Work out the finished part from the listing and answer in its coordinate system (mm). A direction names the side the tool comes from. Round coordinates to 2 decimals unless told otherwise and drop trailing zeros. Write each loop counter-clockwise with the first axis right and the second up, starting at its lowest first coordinate (ties: lowest second). Pieces come first, ordered by that corner, then holes. Notation, with made-up numbers: (9, -21) - (48, -21) arc R20 cw to (48, 17) - close; hole circle Ø4 at (-5, -15). An arc over 180 degrees is marked (long way). Write item = value, one per line. Start each with the question number.
Autodesk Inventor part; units mm, degrees
ref_plane "YZ Plane" through (0, 0, 0) normal (1, 0, 0) x (0, 1, 0)
ref_plane "XZ Plane" through (0, 0, 0) normal (0, 1, 0) x (-1, 0, 0)
ref_plane "XY Plane" through (0, 0, 0) normal (0, 0, 1) x (1, 0, 0)
sketch "Sketch1" plane through (0, 0, 0) normal (1, 0, 0) x (0, 1, 0)
  line L0 (0, 0) -> (44.45, 0)
  line L1 (44.45, 0) -> (44.45, 92.075)
  line L2 (44.45, 92.075) -> (0, 92.075)
  line L3 (0, 92.075) -> (0, 0)
  line L4 (14.2875, 92.075) -> (14.2875, 0) construction
  line L5 (30.1625, 92.075) -> (30.1625, 0) construction
  line L6 (22.225, 92.075) -> (22.225, 0) construction
  circle A0 centre (34.925, 79.375) radius 4.7625 construction
  circle A1 centre (9.525, 12.7) radius 4.7625 construction
  circle A2 centre (34.925, 79.375) radius 7.1437
  circle A3 centre (9.525, 12.7) radius 7.1437
  line L7 (7.9375, 68.2625) -> (36.5125, 68.2625)
  line L8 (36.5125, 68.2625) -> (36.5125, 23.8125)
  line L9 (36.5125, 23.8125) -> (7.9375, 23.8125)
  line L10 (7.9375, 23.8125) -> (7.9375, 68.2625)
  line L11 (7.9375, 46.0375) -> (36.5125, 46.0375) construction
  circle A4 centre (6.0325, 79.375) radius 3.3782
  circle A5 centre (38.4175, 12.7) radius 3.3782
  point P0 (22.225, 68.2625)
  point P1 (22.225, 46.0375)
  dimension "d0" = 15.875
  dimension "d2" = 7.9375
  dimension "d3" = 44.45
  dimension "d4" = 9.525
  dimension "d5" = 9.525
  dimension "d6" = 92.075
  dimension "d7" = 12.7
  dimension "d8" = 12.7
  dimension "d11" = 14.2875
  dimension "d12" = 14.2875
  dimension "d15" = 28.575
  dimension "d16" = 44.45
  dimension "d19" = 6.7564
  dimension "d20" = 6.7564
  dimension "d21" = 8.255
  dimension "d22" = 12.7
  dimension "d23" = 8.255
  dimension "d24" = 12.7
extrude "Extrusion1" add sketch "Sketch1" along normal blind 12.7
fillet "Fillet1" radius 6.35 4 edges at (6.35, 0, 92.075) (6.35, 44.45, 92.075) (6.35, 0, 0) (6.35, 44.45, 0)
fillet "Fillet1" radius 3.175 4 edges at (6.35, 7.9375, 68.2625) (6.35, 36.5125, 68.2625) (6.35, 36.5125, 23.8125) (6.35, 7.9375, 23.8125)
equation "\"d2\" = 0.5 * d0"
equation "\"d23\" = d21"
properties part number "M - Carriage Plate Part 1" material "Aluminum 6061"
1. This flat-tipped pin is pushed along its axis until it touches: pin 1 (18.5 mm diameter, centred on y = 9.525, z = 12.7, fed in from -X). Where does it stop, or does it pass through?
2. Find section B-B on z = 46. Give the vertices of the cut face in (x, y).
3. Find section C-C on z = 12.7. Give the vertices of the cut face in (x, y), plus the area to 3 significant figures.
4. Find section A-A on y = 26.5. Give the vertices of the cut face in (x, z) (1 decimal), plus the area to 3 significant figures.
5. Find section D-D on x = 9.5. Give the number of separate pieces and of enclosed holes in the cut face, plus the area to 3 significant figures.
6. Which of the six approach directions +Z, -Z, +X, -X, +Y, -Y give full straight-line access (tool end or side, diameter ignored) to faces 4 (the face through (6, 22, 92.075)), 5 (the face through (6.439, 35.607, 67.308))?
7. For a pull along Y with two mould halves and no side action, classify faces 1 (the face through (6.439, 1.91, 90.264)), 2 (the face through (6, 22, 68.262)), 3 (the face through (6, 22, 0)) as released by +Y, released by -Y, zero draft, split by the parting line, or undercut.
8. Consider line 1 (Y direction, x = 9.5, z = 60.5); line 2 (Y direction, x = 7.25, z = 82); line 3 (Z direction, x = 1, y = 3.5). Determine where each line is inside the solid, lowest interval first.
Answer key:
q1.pin_1 = 0
q2.outline = (0, 0) - (12.7, 0) - (12.7, 7.94) - (0, 7.94) - close; (0, 36.51) - (12.7, 36.51) - (12.7, 44.45) - (0, 44.45) - close
q3.outline = (0, 0) - (12.7, 0) - (12.7, 2.38) - (0, 2.38) - close; (0, 16.67) - (12.7, 16.67) - (12.7, 35.04) - (0, 35.04) - close; (0, 41.8) - (12.7, 41.8) - (12.7, 44.45) - (0, 44.45) - close
q3.area = 297 mm²
q4.outline = (0, 0) - (12.7, 0) - (12.7, 23.8) - (0, 23.8) - close; (0, 68.3) - (12.7, 68.3) - (12.7, 92.1) - (0, 92.1) - close
q4.area = 605 mm²
q5.separate_pieces = 1
q5.enclosed_holes = 5
q5.area = 2,400 mm²
q6.face_4 = +Z, +X, -X, +Y, -Y
q6.face_5 = +X, -X
q7.face_1 = released by -Y
q7.face_2 = undercut
q7.face_3 = zero draft
q8.line_1 = 0 to 7.94, 36.51 to 44.45
q8.line_2 = 0 to 3.91, 8.16 to 28.28, 41.57 to 44.45
q8.line_3 = 0.68 to 8.86, 16.54 to 77.14, 81.61 to 91.4
